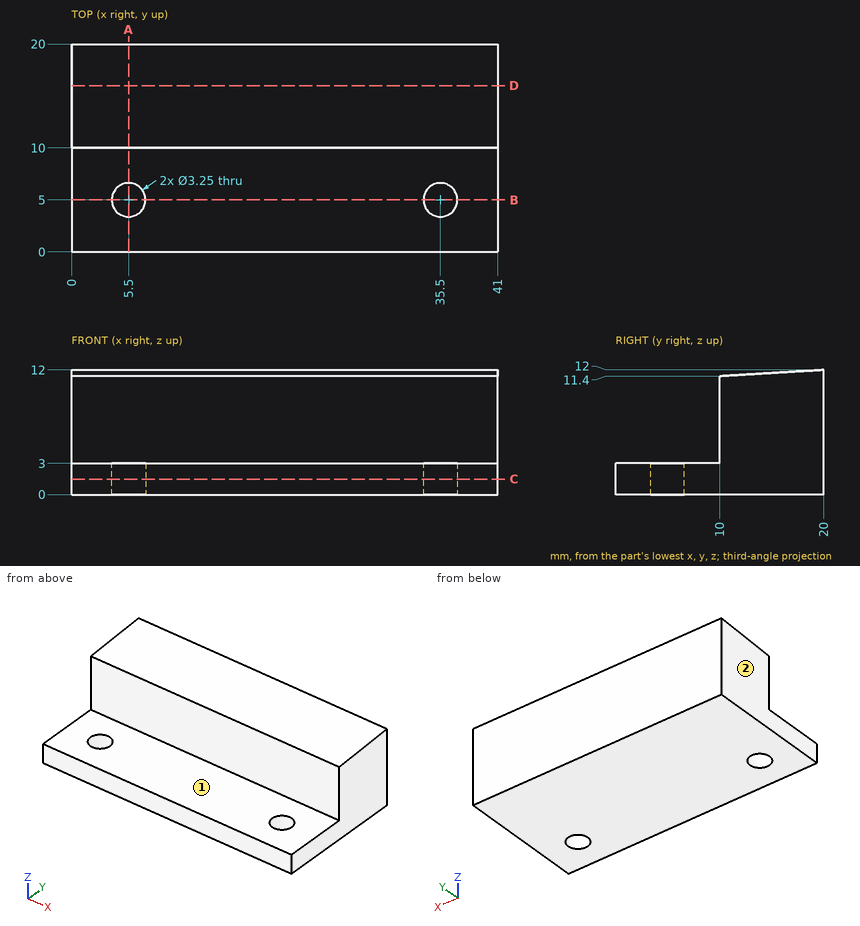
Drawing for the job (mm, zero at the part's lowest x, y, z). A direction names the side the tool comes from. Give positions to 0.01 mm unless a question says otherwise; leave off trailing zeros. Loops run counter-clockwise (first coordinate to the right, second up) from the corner with the lowest first, then second, coordinate; pieces in that order, holes last.
Item 1: Which spindle directions (+Z, -Z, +X, -X, +Y, -Y) get a long thin tool onto all of the face, cutting with end or side? Do the marked faces 1 and 2. Say none if no direction does.
Check values:
face 1: +Z, +X, -X, -Y
face 2: +Z, -Z, -X, +Y, -Y
Item 2: Drill centre lines: line 1 along Y through (x, z) = (35.5, 1.9) (3 decimals); line 2 along Y through (x, z) = (9, 5.75); line 3 along Z through (x, y) = (37.5, 3.5). Where is each one in solid material? Low to high.
Check values:
line 1: y = 0 to 3.375, 6.625 to 20
line 2: y = 10 to 20
line 3: z = 0 to 3
Item 3: Drop flat-ended pins along their axis: P1, Ø4, axis at x = 7, z = 9, coming from the -Y side; P2, Ø11, axis at x = 27, y = 3.5, coming from the +Z side; P3, Ø2.5, axis at x = 35.5, y = 5, coming from the -Z side. Give the stop position or say it passes through.
Check values:
P1: stops at y = 10
P2: stops at z = 3
P3: passes through
Item 4: Slice it at A-A (x = 5.5). Write the cut outline in (y, z) (3 decimals), plus the area to 3 significant figures.
Check values:
outline: (0, 0) - (3.375, 0) - (3.375, 3) - (0, 3) - close; (6.625, 0) - (20, 0) - (20, 12) - (10, 11.4) - (10, 3) - (6.625, 3) - close
area: 137 mm2
Item 5: Slice it at D-D (y = 16). Write the cut outline in (x, z), plus the area to 3 significant figures.
Check values:
outline: (0, 0) - (41, 0) - (41, 11.76) - (0, 11.76) - close
area: 482 mm2
Item 6: Slice it at C-C (z = 1.5). Write the cut outline in (x, y) (3 decimals).
Check values:
outline: (0, 0) - (41, 0) - (41, 20) - (0, 20) - close; hole circle Ø3.25 at (5.5, 5); hole circle Ø3.25 at (35.5, 5)
Item 7: Slice it at B-B (y = 5). Write the cut outline in (x, z) (3 decimals).
Check values:
outline: (0, 0) - (3.875, 0) - (3.875, 3) - (0, 3) - close; (7.125, 0) - (33.875, 0) - (33.875, 3) - (7.125, 3) - close; (37.125, 0) - (41, 0) - (41, 3) - (37.125, 3) - close
